The model under review builds one solid part; all positions refer to its coordinate system, in mm. Face numbers are marked on the shaded views. A direction names the side the tool comes from. Give positions to 0.01 mm unless a question says otherwise; leave off trailing zeros. Loops run counter-clockwise (first coordinate to the right, second up) from the corner with the lowest first, then second, coordinate; pieces in that order, holes last. Notation, with made-up numbers: M -7.5,37 L 44.5,37 A30 cw 44.5,75 Z; hole C 16,-20 d8. An arc over 180 degrees is marked long. Write item = value, one per line. Start each with the question number.
1. For the marked faces 5 and 6, list the 3-axis set-ups (+Z, -Z, +X, -X, +Y, -Y) from which the entire face can be reached by the end or side of a thin tool; tool diameter is ignored.
2. Draft analysis for pull direction Y (two halves, no side actions). For the marked faces 1, 2, 3 and 4, state which applies: pulls with the +Y half, pulls with the -Y half, needs draft (parallel to the pull), parting line crosses it, or undercut.
3. We need section B-B on y = 5.25. Give the boundary of the cut face in (x, z) (3 decimals).
4. Wall thickness on line 1 along X through (y, z) = (8.75, -2.25); line 2 along Y through (x, z) = (-7.15, 0); line 3 along Z through (x, y) = (3, 1.3) (3 decimals): over which ranges is each line inside the solid? List them lowest first. Write a range as from..to.
5. For pin 1 (1.9 mm diameter, centred on y = 9.5, z = 1.5, fed in from -X); pin 2 (1.5 mm diameter, centred on x = 3, z = 0, fed in from +Y), all flat-tipped, find the tip position at first contact; note any pin that passes through.
6. We need section C-C on z = 0. Give the boundary of the cut face in (x, y).
7. We need section A-A on x = -3. Give the boundary of the cut face in (y, z) (3 decimals).
8. We need section D-D on y = 2. Give the boundary of the cut face in (x, z) (3 decimals), then the cut area to 3 significant figures.
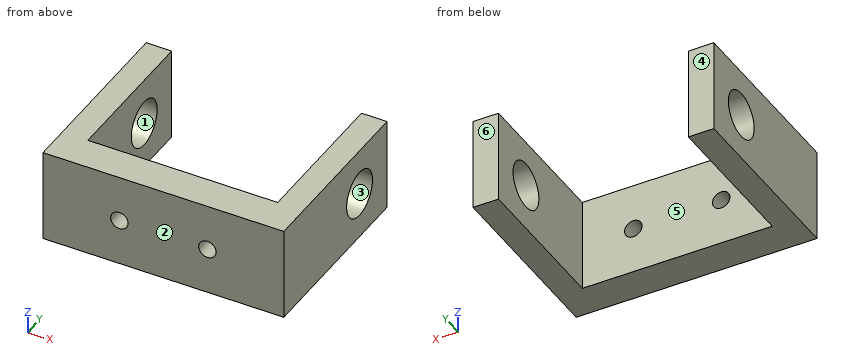
from build123d import *

# Parameters (mm, degrees)
SKETCH1_W             = 16.435294118
SKETCH1_H             = 6.35
BOSS_EXTRUDE1_DEPTH   = 12.7
SKETCH2_W             = 12.954
SKETCH2_H             = 6.35
CUT_EXTRUDE1_DEPTH    = 10.31875
SKETCH3_R             = 1.5875
CUT_EXTRUDE2_DEPTH    = 17.435294118
F_0_80_TAPPED_HOLE1_D = 1.19126


with BuildPart() as part:
    # Sketch1 → Boss-Extrude1 (new body)
    with BuildSketch(Plane(origin=(0, 0, 0), x_dir=(1, 0, 0), z_dir=(0, 1, 0))):
        Rectangle(SKETCH1_W, SKETCH1_H)
    extrude(amount=BOSS_EXTRUDE1_DEPTH)

    # Sketch2 → Cut-Extrude1 (cut)
    with BuildSketch(Plane(origin=(0, 12.7, 0), x_dir=(-1, 0, 0), z_dir=(0, 1, 0))):
        Rectangle(SKETCH2_W, SKETCH2_H)
    extrude(amount=-CUT_EXTRUDE1_DEPTH, mode=Mode.SUBTRACT)

    # Sketch3 → Cut-Extrude2 (cut, through all)
    with BuildSketch(Plane(origin=(8.217647059, 0, 0), x_dir=(0, 0, -1), z_dir=(1, 0, 0))):
        with Locations((0, 9.3218)):
            Circle(SKETCH3_R)
    extrude(amount=-CUT_EXTRUDE2_DEPTH, mode=Mode.SUBTRACT)

    # #0-80 Tapped Hole1 (through all)
    with Locations(Plane(origin=(0, 2.38125, 0), x_dir=(-1, 0, 0), z_dir=(0, 1, 0))):
        with Locations((3, 0), (-3, 0)):
            Hole(F_0_80_TAPPED_HOLE1_D / 2)


solid = part.part
Final values:
q1.face_5 = +Z, -Z, +Y
q1.face_6 = +Z, -Z, +X, -X, +Y
q2.face_1 = undercut
q2.face_2 = pulls with the -Y half
q2.face_3 = undercut
q2.face_4 = pulls with the +Y half
q3.outline = M -8.218,-3.175 L -6.477,-3.175 L -6.477,3.175 L -8.218,3.175 Z; M 6.477,-3.175 L 8.218,-3.175 L 8.218,3.175 L 6.477,3.175 Z
q4.line_1 = -8.22..-6.48, 6.48..8.22
q4.line_2 = 0..7.73, 10.91..12.7
q4.line_3 = -3.175..-0.596, 0.596..3.175
q5.pin_1 = -8.22
q5.pin_2 = 2.38
q6.outline = M -8.22,0 L -3.6,0 L -3.6,2.38 L -6.48,2.38 L -6.48,7.73 L -8.22,7.73 Z; M -8.22,10.91 L -6.48,10.91 L -6.48,12.7 L -8.22,12.7 Z; M -2.4,0 L 2.4,0 L 2.4,2.38 L -2.4,2.38 Z; M 3.6,0 L 8.22,0 L 8.22,7.73 L 6.48,7.73 L 6.48,2.38 L 3.6,2.38 Z; M 6.48,10.91 L 8.22,10.91 L 8.22,12.7 L 6.48,12.7 Z
q7.outline = M 0,-3.175 L 2.381,-3.175 L 2.381,-0.596 L 0,-0.596 Z; M 0,0.596 L 2.381,0.596 L 2.381,3.175 L 0,3.175 Z
q8.outline = M -8.218,-3.175 L 8.218,-3.175 L 8.218,3.175 L -8.218,3.175 Z; hole C -3,0 d1.191; hole C 3,0 d1.191
q8.area = 102 mm²
